```python
from build123d import *

# Parameters (mm, degrees)
ESQUISSE1_W             = 17.2
ESQUISSE1_H             = 22.6
BOSS_EXTRU_1_DEPTH      = 6.2
ENL_V_MAT_EXTRU_1_DEPTH = 3.8
ESQUISSE3_R             = 0.9
ENL_V_MAT_EXTRU_2_DEPTH = 25.477744994
CHANFREIN1_SIZE         = 2
BOSS_EXTRU_2_DEPTH      = 18.6
BOSS_EXTRU_3_DEPTH      = 4
CONG_1_R                = 2


with BuildPart() as part:
    # Esquisse1 → Boss.-Extru.1 (new body)
    with BuildSketch(Plane(origin=(0, 0, 0), x_dir=(1, 0, 0), z_dir=(0, 1, 0))):
        with Locations((0, 11.3)):
            Rectangle(ESQUISSE1_W, ESQUISSE1_H)
    extrude(amount=BOSS_EXTRU_1_DEPTH)

    # Esquisse2 → Enlèv. mat.-Extru.1 (cut)
    with BuildSketch(Plane(origin=(0, 6.2, 0), x_dir=(1, 0, 0), z_dir=(0, 1, 0))):
        with BuildLine():
            Line((-5.1, 4), (5.1, 4))
            Line((5.1, 4), (6.1, 5))
            Line((6.1, 5), (6.1, 6.8))
            ThreePointArc((6.1, 6.8), (7, 7.7), (6.1, 8.6))
            Line((6.1, 8.6), (6.1, 11.6))
            ThreePointArc((6.1, 11.6), (7, 12.5), (6.1, 13.4))
            Line((6.1, 13.4), (6.1, 15.2))
            Line((6.1, 15.2), (5.1, 16.2))
            Line((5.1, 16.2), (-5.1, 16.2))
            Line((-5.1, 16.2), (-6.1, 15.2))
            Line((-6.1, 15.2), (-6.1, 13.4))
            ThreePointArc((-6.1, 13.4), (-7, 12.5), (-6.1, 11.6))
            Line((-6.1, 11.6), (-6.1, 8.6))
            ThreePointArc((-6.1, 8.6), (-7, 7.7), (-6.1, 6.8))
            Line((-6.1, 6.8), (-6.1, 5))
            Line((-6.1, 5), (-5.1, 4))
        make_face()
    extrude(amount=-ENL_V_MAT_EXTRU_1_DEPTH, mode=Mode.SUBTRACT)

    # Esquisse3 → Enlèv. mat.-Extru.2 (cut, through all)
    with BuildSketch(Plane(origin=(0, 2.4, 0), x_dir=(1, 0, 0), z_dir=(0, 1, 0))):
        with Locations(Location((6.1, 12.5, 0), (0, 0, 270))):
            Circle(ESQUISSE3_R)
        with Locations(Location((-6.1, 12.5, 0), (0, 0, 270))):
            Circle(ESQUISSE3_R)
        with Locations(Location((-6.1, 7.7, 0), (0, 0, 270))):
            Circle(ESQUISSE3_R)
        with Locations(Location((6.1, 7.7, 0), (0, 0, 270))):
            Circle(ESQUISSE3_R)
    extrude(amount=-ENL_V_MAT_EXTRU_2_DEPTH, mode=Mode.SUBTRACT)

    # Chanfrein1
    # the kernel refuses this chamfer: 2 mm, written as the material it takes off along each edge
    with BuildSketch(Plane(origin=(13.743365976, 0, -22.6), x_dir=(0, -0.02749587661058639, 0.9996219169112968), z_dir=(-1, 0, 0))) as chanfrein1_piece_1:
        Polygon((CHANFREIN1_SIZE * 0.999621916911, CHANFREIN1_SIZE * 0.0274958766106), (-CHANFREIN1_SIZE * 0.0274958766106, CHANFREIN1_SIZE * 0.999621916911), (0, 0), align=None)
    extrude(amount=27.486731952, mode=Mode.SUBTRACT)
    with BuildSketch(Plane(origin=(8.6, 0, 5.143365976), x_dir=(0.027495876610586494, 0.9996219169112968, 0), z_dir=(0, 0, -1)), Plane(origin=(-8.6, 0, -27.743365976), x_dir=(-0.027495876610586494, 0.9996219169112968, 0), z_dir=(0, 0, 1))) as chanfrein1_piece_2:
        Polygon((CHANFREIN1_SIZE * 0.999621916911, -CHANFREIN1_SIZE * 0.0274958766106), (-CHANFREIN1_SIZE * 0.0274958766106, -CHANFREIN1_SIZE * 0.999621916911), (0, 0), align=None)
    extrude(amount=32.886731952, mode=Mode.SUBTRACT)

    # Esquisse4 → Boss.-Extru.2 (add)
    with BuildSketch(Plane(origin=(0, 0, -22.6), x_dir=(-1, 0, 0), z_dir=(0, 0, -1))):
        with BuildLine():
            Line((-8.6, 6.2), (-8.6, 5.2))
            ThreePointArc((-8.6, 5.2), (-12.321519298, 6.230801171), (-14.982352941, 9.029411765))
            Line((-14.982352941, 9.029411765), (-14.982352941, 9.5))
            Line((-14.982352941, 9.5), (-14.1, 9.5))
            ThreePointArc((-14.1, 9.5), (-11.807023542, 7.088294096), (-8.6, 6.2))
        make_face()
    boss_extru_2 = extrude(amount=-BOSS_EXTRU_2_DEPTH)

    # Symétrie1: Boss.-Extru.2 across plane
    add(boss_extru_2.mirror(Plane(origin=(0, 0, 0), x_dir=(0, 0, 1), z_dir=(1, 0, 0))))

    # Esquisse5 → Boss.-Extru.3 (add, symmetric)
    with BuildSketch(Plane(origin=(0, 0, 0), x_dir=(0, 0, -1), z_dir=(1, 0, 0))):
        Polygon((4, 0), (8, 0), (5, -3), (4, -3), align=None)
    extrude(amount=BOSS_EXTRU_3_DEPTH, both=True)

    # Congé1
    cong_1_edges = [part.edges().sort_by_distance(p)[0] for p in [
        (8.6, 5.2, -13.3),
        (-8.6, 5.2, -13.3),
        (0, 0, -8),
    ]]
    fillet(cong_1_edges, radius=CONG_1_R)


solid = part.part
```
For this review, take the finished solid that the model builds, in its own axes (mm). A direction names the side the tool comes from. Round coordinates to 2 decimals unless told otherwise and drop trailing zeros. Loops run counter-clockwise (first coordinate to the right, second up) from the corner with the lowest first, then second, coordinate; pieces in that order, holes last.
Q1. Add section D-D on y = 3. Write out the cut boundary in (x, z).
Result sheet:
outline: (-8.6, -22.6) - (8.6, -22.6) - (8.6, 0) - (-8.6, 0) - close; hole (-6.1, -15.2) - (-5.1, -16.2) - (5.1, -16.2) - (6.1, -15.2) - (6.1, -13.4) arc R0.9 ccw to (6.1, -11.6) - (6.1, -8.6) arc R0.9 ccw to (6.1, -6.8) - (6.1, -5) - (5.1, -4) - (-5.1, -4) - (-6.1, -5) - (-6.1, -6.8) arc R0.9 ccw to (-6.1, -8.6) - (-6.1, -11.6) arc R0.9 ccw to (-6.1, -13.4) - close
Q2. Add section B-B on y = 1.5. Write out the cut boundary in (x, z).
Result sheet:
outline: (-8.1, -22.1) - (8.1, -22.1) - (8.1, 0) - (-8.1, 0) - close; hole circle Ø1.8 at (-6.1, -12.5); hole circle Ø1.8 at (-6.1, -7.7); hole circle Ø1.8 at (6.1, -12.5); hole circle Ø1.8 at (6.1, -7.7)
Q3. To check wall thickness, follow line 1 along X through (y, z) = (2, -7.7); line 2 along Z through (x, y) = (-6.1, 2); line 3 along X through (y, z) = (1.5, -12.5). State the ranges of each line that lie inside material, in increasing order.
Result sheet:
line 1: x = -8.6 to -7, -5.2 to 5.2, 7 to 8.6
line 2: z = -22.6 to -13.4, -11.6 to -8.6, -6.8 to 0
line 3: x = -8.1 to -7, -5.2 to 5.2, 7 to 8.1
Q4. Insertion check: pin 1 Ø2.5 at (x, z) = (6.1, -12.5) entering from +Y; pin 2 Ø6 at (y, z) = (2, -5) entering from +X; pin 3 Ø2 at (y, z) = (3.5, -6) entering from -X. Each pin has a flat end and moves straight along its axis. Give the tip position at first contact, or say it passes through.
Result sheet:
pin 1: stops at y = 6.2
pin 2: stops at x = 9.37
pin 3: stops at x = -8.92
Q5. Add section A-A on z = -12.5. Write out the cut boundary in (x, y).
Result sheet:
outline: (-14.98, 9.03) arc R7.23 ccw to (-10.17, 5.37) arc R2 cw to (-8.6, 3.42) - (-8.6, 2) - (-7, 0.4) - (-7, 6.2) - (-8.6, 6.2) arc R6.23 cw to (-14.1, 9.5) - (-14.98, 9.5) - close; (-5.2, 0) - (5.2, 0) - (5.2, 2.4) - (-5.2, 2.4) - close; (7, 0.4) - (8.6, 2) - (8.6, 3.42) arc R2 cw to (10.17, 5.37) arc R7.23 ccw to (14.98, 9.03) - (14.98, 9.5) - (14.1, 9.5) arc R6.23 cw to (8.6, 6.2) - (7, 6.2) - close
Q6. Mouldability with a two-part tool opening along Z and no side actions: class faces 1 (the face through (-7, 2.45, -7.76)), 2 (the face through (0, -2, -4)), 3 (the face through (14.5, 9.5, -13.4)) as +Z half, -Z half, draft (parallel to the pull), parting line (faces both ways), or undercut.
Result sheet:
face 1: undercut
face 2: +Z half
face 3: draft
Q7. Machinability: for faces 4 (the face through (6.1, 4, -6)), 5 (the face through (-4, -1, -5)), 6 (the face through (8.6, 3, -9)), 7 (the face through (-11.847, 7.113, -13.43)), 8 (the face through (-12, 7, -4)), which of the approach directions +Z, -Z, +X, -X, +Y, -Y give a long, thin tool a straight path to every point of the face, cutting with its end or side? Answer none if there is none.
Result sheet:
face 4: +Y
face 5: +Z, -Z, -X, -Y
face 6: +Z, +X, -Y
face 7: +Z, -Z, +Y
face 8: +Z, -X, +Y, -Y
Q8. Add section C-C on x = -4.5. Write out the cut boundary in (y, z).
Result sheet:
outline: (0, -20.6) - (2, -22.6) - (6.2, -22.6) - (6.2, -16.2) - (2.4, -16.2) - (2.4, -4) - (6.2, -4) - (6.2, 0) - (0, 0) - close
